Read the model definition and answer for the solid it produces. Units are mm, in the model's axes. Face numbers are marked on the shaded views. A direction names the side the tool comes from. Round coordinates to 2 decimals unless told otherwise and drop trailing zeros. Order: outer loops, then holes, each group sorted by start corner. A loop starts at its lowest first (then second) coordinate and runs counter-clockwise, first axis right, second up. Notation, with made-up numbers: M -31,-36 L 12,-36 A16 cw 12,-13 Z; hole C 16,32 d6. An arc over 180 degrees is marked long. Answer as CSV lines item,"result".
```python
from build123d import *

# Parameters (mm, degrees)
SKETCH105_W     = 73.9
SKETCH105_H     = 3
PAD050_DEPTH    = 73.9
SKETCH108_R     = 1
PAD052_DEPTH    = 3
SKETCH109_W     = 70.9
SKETCH109_H     = 2
PAD053_DEPTH    = 2
SKETCH110_R     = 2.6
PAD056_DEPTH    = 35
SKETCH111_R     = 1.05
POCKET060_DEPTH = 8
PAD060_START    = 3.9
SKETCH125_R     = 17.5
PAD060_DEPTH    = 66.1
SKETCH126_R     = 16
SKETCH126_W     = 30
SKETCH126_H     = 12
POCKET075_DEPTH = 73.901
PAD061_START    = 3.9
SKETCH127_W     = 15
SKETCH127_H     = 2
PAD061_DEPTH    = 66.1
SKETCH128_R     = 2.1
POCKET076_DEPTH = 73.901
SKETCH129_R     = 1
POCKET077_DEPTH = 5


with BuildPart() as part:
    # Sketch105 → Pad050 (new body)
    with BuildSketch(Plane.XY):
        with Locations((36.95, 1.5)):
            Rectangle(SKETCH105_W, SKETCH105_H)
    extrude(amount=PAD050_DEPTH)

    # Sketch108 → Pad052 (join)
    with BuildSketch(Plane.YZ):
        with BuildLine():
            Line((3, 0), (80, 0))
            ThreePointArc((80, 0), (89.1923881554, 3.8076118446), (93, 13))
            Line((93, 13), (93, 60.9))
            ThreePointArc((93, 60.9), (89.1923881554, 70.0923881554), (80, 73.9))
            Line((80, 73.9), (3, 73.9))
            Line((3, 73.9), (3, 0))
        make_face()
        with Locations((7, 2)):
            Circle(SKETCH108_R, mode=Mode.SUBTRACT)
        with Locations((74, 2)):
            Circle(SKETCH108_R, mode=Mode.SUBTRACT)
        with Locations((7, 71.9)):
            Circle(SKETCH108_R, mode=Mode.SUBTRACT)
        with Locations((74, 71.9)):
            Circle(SKETCH108_R, mode=Mode.SUBTRACT)
    extrude(amount=PAD052_DEPTH)

    # Sketch109 → Pad053 (join)
    with BuildSketch(Plane(origin=(0, 3, 0), x_dir=(-1, 0, 0), z_dir=(0, 1, 0))):
        with Locations((-38.45, 2)):
            Rectangle(SKETCH109_W, SKETCH109_H)
        with Locations((-38.45, 71.9)):
            Rectangle(SKETCH109_W, SKETCH109_H)
    extrude(amount=PAD053_DEPTH)

    # Sketch110 → Pad056 (join)
    with BuildSketch(Plane.YZ):
        with Locations((72, 14.45)):
            Circle(SKETCH110_R)
        with Locations((8, 14.45)):
            Circle(SKETCH110_R)
        with Locations((8, 59.45)):
            Circle(SKETCH110_R)
        with Locations((72, 59.45)):
            Circle(SKETCH110_R)
    extrude(amount=PAD056_DEPTH)

    # Sketch111 → Pocket060 (cut)
    with BuildSketch(Plane.YZ.offset(35)):
        with Locations((8, 14.45)):
            Circle(SKETCH111_R)
        with Locations((72, 14.45)):
            Circle(SKETCH111_R)
        with Locations((8, 59.45)):
            Circle(SKETCH111_R)
        with Locations((72, 59.45)):
            Circle(SKETCH111_R)
    extrude(amount=-POCKET060_DEPTH, mode=Mode.SUBTRACT)

    # Sketch125 → Pad060 (join)
    with BuildSketch(Plane.YZ.offset(PAD060_START)):
        with Locations((-17, 36.95)):
            Circle(SKETCH125_R)
    extrude(amount=PAD060_DEPTH)

    # Sketch126 → Pocket075 (cut, through all)
    with BuildSketch(Plane.YZ):
        with Locations((-17, 36.95)):
            Circle(SKETCH126_R)
        with Locations((-27.180588, 36.95)):
            Rectangle(SKETCH126_W, SKETCH126_H)
    extrude(amount=POCKET075_DEPTH, mode=Mode.SUBTRACT)

    # Sketch127 → Pad061 (join)
    with BuildSketch(Plane.YZ.offset(PAD061_START)):
        with Locations((-39.5, 43.95)):
            Rectangle(SKETCH127_W, SKETCH127_H)
        with Locations((-39.5, 29.95)):
            Rectangle(SKETCH127_W, SKETCH127_H)
    extrude(amount=PAD061_DEPTH)

    # Sketch128 → Pocket076 (cut, through all)
    with BuildSketch(Plane.XY):
        with Locations((9.9, -41.5)):
            Circle(SKETCH128_R)
        with Locations((64.9, -41.5)):
            Circle(SKETCH128_R)
    extrude(amount=POCKET076_DEPTH, mode=Mode.SUBTRACT)

    # Sketch129 → Pocket077 (cut)
    with BuildSketch(Plane.XZ):
        with Locations((70.9, 10)):
            Circle(SKETCH129_R)
        with Locations((70.9, 63.9)):
            Circle(SKETCH129_R)
    extrude(amount=-POCKET077_DEPTH, mode=Mode.SUBTRACT)


solid = part.part
```
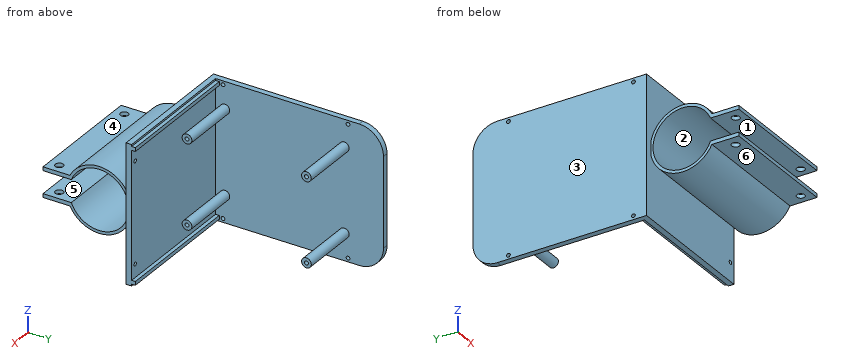
Item 1: A cutting plane is placed at D-D, the plane y = -23. Determine the outline of the cut face in (x, z).
Ans:
outline,"M 3.9,20.51 L 70,20.51 L 70,22.12 L 3.9,22.12 Z; M 3.9,51.78 L 70,51.78 L 70,53.39 L 3.9,53.39 Z"
Item 2: Find the intervals of material crossed by probe 1 along Z at (x, y) = (1.05, 74); probe 2 along Y at (x, z) = (1.45, 71.9); probe 3 along Y at (x, z) = (15.5, 29), in increasing order. Write a range as [from, to].
Ans:
probe 1,"[0, 1], [3, 70.9], [72.9, 73.9]"
probe 2,"[0, 6], [8, 73], [75, 86.93]"
probe 3,"[-47, -30.89], [-3.11, -1.41], [0, 3]"
Item 3: Flat-ended cylindrical pins translate along their axes: pin 1 (1.5 mm diameter, centred on x = 37, z = 53, fed in from +Y); pin 2 (1 mm diameter, centred on x = 30.5, y = 4, fed in from +Z); pin 3 (1 mm diameter, centred on x = 46.5, z = 16.5, fed in from -Y). Find the tip coordinate at first contact, or state that the pin passes through.
Ans:
pin 1,"y = 3"
pin 2,"z = 72.9"
pin 3,"y = 0"
Item 4: A cutting plane is placed at A-A, the plane x = 9.9. Give the number of separate pieces and of enclosed holes in the cut face, and give its area (3 significant figures).
Ans:
separate pieces,"7"
enclosed holes,"0"
area,"490 mm2"
Item 5: A tool of negligible diameter and unlimited length cuts with its end or side. For the marked faces 5 and 6, from which of +Z, -Z, +X, -X, +Y, -Y can it reach the whole face along a straight path? Write none if from no direction.
Ans:
face 5,"+X, -X, -Y"
face 6,"-Z, +X, -X, -Y"
Item 6: A cutting plane is placed at B-B, the plane y = -41.5. Determine the outline of the cut face in (x, z), and give its area (3 significant figures).
Ans:
outline,"M 3.9,28.95 L 7.8,28.95 L 7.8,30.95 L 3.9,30.95 Z; M 3.9,42.95 L 7.8,42.95 L 7.8,44.95 L 3.9,44.95 Z; M 12,28.95 L 62.8,28.95 L 62.8,30.95 L 12,30.95 Z; M 12,42.95 L 62.8,42.95 L 62.8,44.95 L 12,44.95 Z; M 67,28.95 L 70,28.95 L 70,30.95 L 67,30.95 Z; M 67,42.95 L 70,42.95 L 70,44.95 L 67,44.95 Z"
area,"231 mm2"
Item 7: Determine the mould class of the marked faces 1, 2, 3 and 4 for opening direction Z: +Z half, -Z half, draft (parallel to the pull), parting line (faces both ways), or undercut.
Ans:
face 1,"undercut"
face 2,"undercut"
face 3,"draft"
face 4,"+Z half"
